from build123d import *

# Parameters (mm, degrees)
F0_R     = 11.0109
F1_DEPTH = 7.747


with BuildPart() as f1:
    # F0 (on Top) → F1 (new body)
    with BuildSketch(Plane.XY):
        with BuildLine():
            Line((5.30555, 13.096203), (10.931762, 18.253563))
            ThreePointArc((10.931762, 18.253563), (7.899724, 38.408908), (-12.041939, 34.194499))
            ThreePointArc((-12.041939, 34.194499), (-18.394659, 16.410973), (-13.994419, -1.953361))
            Line((-13.994419, -1.953361), (-21.27393, 0.340402))
            ThreePointArc((-21.27393, 0.340402), (-37.212952, -12.363092), (-23.592335, -27.525875))
            ThreePointArc((-23.592335, -27.525875), (-5.01499, -24.135728), (8.68887, -11.142842))
            Line((8.68887, -11.142842), (10.342168, -18.593965))
            ThreePointArc((10.342168, -18.593965), (29.313228, -26.045816), (35.634275, -6.668624))
            ThreePointArc((35.634275, -6.668624), (23.409649, 7.724756), (5.30555, 13.096203))
        make_face()
        with Locations((-23.255562, -13.524312)):
            Circle(F0_R, mode=Mode.SUBTRACT)
        Polygon((-3.755629, -14.376059), (-3.755629, -20.868891), (-9.378587, -17.622475), align=None, mode=Mode.SUBTRACT)
        Circle(F0_R, mode=Mode.SUBTRACT)
        with Locations((23.340179, -13.377751)):
            Circle(F0_R, mode=Mode.SUBTRACT)
        Polygon((14.327847, 3.935559), (19.950804, 7.181975), (19.950804, 0.689143), align=None, mode=Mode.SUBTRACT)
        Polygon((-16.195175, 13.686916), (-10.572217, 16.933332), (-10.572217, 10.4405), align=None, mode=Mode.SUBTRACT)
        with Locations((0, 26.692882)):
            Circle(F0_R, mode=Mode.SUBTRACT)
    extrude(amount=F1_DEPTH)


solid = f1.part
Check sheet for the modelled part. Datum: model origin and axes. Units: mm. A direction names the side the tool comes from. Round coordinates to 2 decimals unless told otherwise and drop trailing zeros. Loops run counter-clockwise (first coordinate to the right, second up) from the corner with the lowest first, then second, coordinate; pieces in that order, holes last. Notation, with made-up numbers: M -37.5,3.5 L -9.5,3.5 A11 cw -9.5,19.5 Z; hole C 17,45 d4. An arc over 180 degrees is marked long. One line per item, written item: value.
(1) Sectioned sample at C-C, the plane z = 2. Record the cut outline in (x, y).
Computed values:
outline: M -23.59,-27.53 A33.12 ccw 8.69,-11.14 L 10.34,-18.59 A14.01 ccw long 35.63,-6.67 A33.12 ccw 5.31,13.1 L 10.93,18.25 A14.01 ccw long -12.04,34.19 A33.12 ccw -13.99,-1.95 L -21.27,0.34 A14.01 ccw long Z; hole C -23.26,-13.52 d22.02; hole M -16.2,13.69 L -10.57,10.44 L -10.57,16.93 Z; hole C 0,0 d22.02; hole C 0,26.69 d22.02; hole M -9.38,-17.62 L -3.76,-20.87 L -3.76,-14.38 Z; hole C 23.34,-13.38 d22.02; hole M 14.33,3.94 L 19.95,0.69 L 19.95,7.18 Z
(2) Access from +Z, -Z, +X, -X, +Y, -Y to the whole of each face (thin tool, end or side, straight path). Record for faces 5 (the face through (-11, 2, 7.747)), 6 (the face through (19.951, 4, 4)).
Computed values:
face 5: +Z, +X, -X, +Y, -Y
face 6: +Z, -Z
(3) Depth check by flat-ended pin: pin 1 Ø4 at (y, z) = (20.5, 2.5) entering from +X; pin 2 Ø1.5 at (y, z) = (17.5, 2) entering from -X; pin 3 Ø2 at (y, z) = (3.5, 5.5) entering from -X. Enter the tip coordinate at first touch or a pass-through.
Computed values:
pin 1: stops at x = 13.21
pin 2: stops at x = -18.37
pin 3: stops at x = -16.86
(4) Sectioned sample at B-B, the plane y = -9. Record the cut outline in (x, z), then the cut area to 3 significant figures.
Computed values:
outline: M -36.51,0 L -33.29,0 L -33.29,7.75 L -36.51,7.75 Z; M -13.22,0 L -6.34,0 L -6.34,7.75 L -13.22,7.75 Z; M 6.34,0 L 13.24,0 L 13.24,7.75 L 6.34,7.75 Z; M 33.44,0 L 36.64,0 L 36.64,7.75 L 33.44,7.75 Z
area: 156 mm^2
(5) Release check for a two-part mould opening along X. For faces 1 (the face through (-11, 2, 0)), 2 (the face through (10.502, 30, 3.819)), 3 (the face through (-17.583, -0.823, 3.819)), 4 (the face through (8.08, 15.64, 3.82)) record: +X half, -X half, draft (parallel to the pull), parting line (faces both ways), or undercut.
Computed values:
face 1: draft
face 2: undercut
face 3: undercut
face 4: +X half
(6) Thickness scan on line 1 (X direction, y = -18, z = 6); line 2 (Y direction, x = -2.5, z = 6.5); line 3 (Y direction, x = 3.5, z = 1.75). Record the ranges inside material, lowest first.
Computed values:
line 1: x = -36.53 to -33.32, -13.2 to -8.72, -3.76 to 3.44, 10.21 to 13.35, 33.33 to 36.56
line 2: y = -22.72 to -10.72, 10.72 to 15.97, 37.42 to 40.7
line 3: y = -17.94 to -10.44, 10.44 to 16.25, 37.13 to 40.44
(7) Sectioned sample at A-A, the plane x = 3. Record the cut outline in (y, z), then the cut area to 3 significant figures.
Computed values:
outline: M -18.43,0 L -10.59,0 L -10.59,7.75 L -18.43,7.75 Z; M 10.59,0 L 16.1,0 L 16.1,7.75 L 10.59,7.75 Z; M 37.29,0 L 40.56,0 L 40.56,7.75 L 37.29,7.75 Z
area: 129 mm^2
(8) Sectioned sample at D-D, the plane y = 25.5. Record the cut outline in (x, z).
Computed values:
outline: M -16.61,0 L -10.95,0 L -10.95,7.75 L -16.61,7.75 Z; M 10.95,0 L 13.85,0 L 13.85,7.75 L 10.95,7.75 Z
